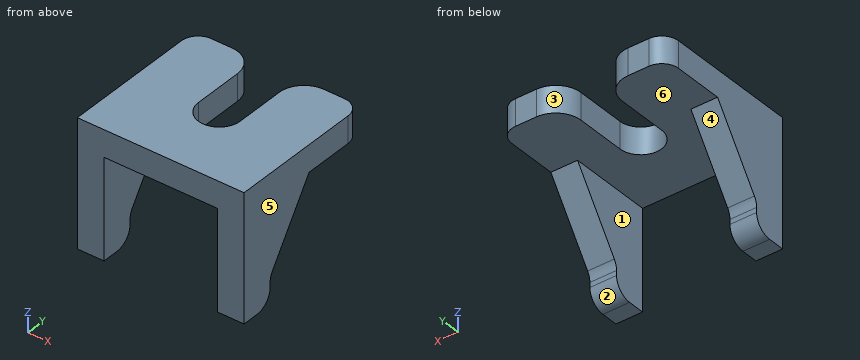
```python
from build123d import *

# Parameters (mm, degrees)
PAD006_DEPTH            = 1.6
PAD007_DEPTH            = 1.6
LINEARPATTERN009_COUNT  = 2
LINEARPATTERN009_PITCH  = 8.4
FILLET008_R             = 1
FILLET009_R             = 1
FILLET035_R             = 1
FILLET036_R             = 1.5
BODY003_PLACEMENT_ANGLE = 90


with BuildPart() as part:
    # Sketch110 → Pad006 (new body)
    with BuildSketch(Plane.XY):
        with BuildLine():
            Line((-4.5, 5), (4.5, 5))
            Line((4.5, 5), (4.5, 1.25))
            Line((0, 1.25), (4.5, 1.25))
            ThreePointArc((0, 1.25), (-1.25, 0), (0, -1.25))
            Line((4.5, -1.25), (0, -1.25))
            Line((4.5, -1.25), (4.5, -5))
            Line((4.5, -5), (-4.5, -5))
            Line((-4.5, -5), (-4.5, 5))
        make_face()
    extrude(amount=PAD006_DEPTH)

    # Sketch111 (on DatumPlane) → Pad007 (join)
    with BuildSketch(Plane.XZ.offset(5)):
        Polygon((-4.5, 0), (-4.5, -6), (-2.5, -6), (-2.5, -4.4), (0.5, 0), align=None)
    pad007 = extrude(amount=-PAD007_DEPTH)

    # LinearPattern009: Pad007 ×2
    with Locations(*[(0, i * LINEARPATTERN009_PITCH, 0) for i in range(1, LINEARPATTERN009_COUNT)]):
        add(pad007)

    # Fillet008
    fillet008_edges = [part.edges().sort_by_distance(p)[0] for p in [
        (-2.5, -4.2, -6),
        (-2.5, 4.2, -6),
    ]]
    fillet(fillet008_edges, radius=FILLET008_R)

    # Fillet009
    fillet009_edges = [part.edges().sort_by_distance(p)[0] for p in [
        (-2.5, -4.2, -4.4),
        (-2.5, 4.2, -4.4),
    ]]
    fillet(fillet009_edges, radius=FILLET009_R)

    # Fillet035
    fillet035_edges = [part.edges().sort_by_distance(p)[0] for p in [
        (4.5, -5, 0.8),
        (4.5, 5, 0.8),
    ]]
    fillet(fillet035_edges, radius=FILLET035_R)

    # Fillet036
    fillet036_edges = [part.edges().sort_by_distance(p)[0] for p in [
        (4.5, -1.25, 0.8),
        (4.5, 1.25, 0.8),
    ]]
    fillet(fillet036_edges, radius=FILLET036_R)


with BuildPart() as part_1:
    # Body003 placement: moved
    add(part.part.moved(Location((-22.4, 32.5, 16.4))).rotate(Axis((-22.4, 32.5, 16.4), (0, 0, 1)), BODY003_PLACEMENT_ANGLE))


solid = part_1.part
```
Input: part model. Units: mm. Frame: model coordinates. Face numbers are marked on the shaded views. A direction names the side the tool comes from. Give positions to 0.01 mm unless a question says otherwise; leave off trailing zeros. Order: outer loops, then holes, each group sorted by start corner. A loop starts at its lowest first (then second) coordinate and runs counter-clockwise, first axis right, second up. Notation, with made-up numbers: M 85,-8.5 L 115,-8.5 A31 cw 115,22.5 Z; hole C -25.5,22 d5. An arc over 180 degrees is marked long. One line per question, with ' | ' between items.
1) Access query for the marked faces 1, 2 and 3. Directions: +Z, -Z, +X, -X, +Y, -Y. A direction counts if a zero-diameter tool reaches every point of the face in a straight line with its end or side. Return the directions, or none.
Filled in:
face 1: -Z, +Y, -Y | face 2: -Z, +X, -X, +Y | face 3: +Z, -Z, +Y
2) Section A-A on y = 33.5. Output: boundary loops of the cut face in (x, z), and give its area (3 significant figures).
Filled in:
outline: M -27.4,16.4 L -23.65,16.4 L -23.65,18 L -27.4,18 Z; M -21.15,16.4 L -17.4,16.4 L -17.4,18 L -21.15,18 Z | area: 12.0 mm2
3) Section D-D on y = 29.25. Output: boundary loops of the cut face in (x, z), and give its area (3 significant figures).
Filled in:
outline: M -27.4,10.43 L -25.8,10.43 L -25.8,16.4 L -19,16.4 L -19,10.43 L -17.4,10.43 L -17.4,18 L -27.4,18 Z | area: 35.1 mm2
4) Contact query for flat-ended pins moving along their axis: P1, Ø4, axis at x = -19.5, y = 34, coming from the -Z side; P2, Ø4, axis at y = 31, z = 13, coming from the -X side; P3, Ø3, axis at x = -24, z = 13.5, coming from the -Y side. Output: stop coordinate, or through.
Filled in:
P1: stops at z = 15.03 | P2: stops at x = -27.4 | P3: passes through
5) Draft query along X for the marked faces 4, 5 and 6. Return one class per face: pulls with the +X half, pulls with the -X half, needs draft (parallel to the pull), parting line crosses it, or undercut.
Filled in:
face 4: needs draft | face 5: pulls with the +X half | face 6: undercut
6) Ray query, L1, parallel to X at y = 30, z = 15; L2, parallel to Z at x = -20.25, y = 33; L3, parallel to X at y = 32.25, z = 17.5. Return the intervals inside material, ascending.
Filled in:
L1: x = -27.4 to -25.8, -19 to -17.4 | L2: z = 16.4 to 18 | L3: x = -27.4 to -23.62, -21.18 to -17.4
7) Section C-C on z = 17.25. Output: boundary loops of the cut face in (x, y).
Filled in:
outline: M -27.4,28 L -17.4,28 L -17.4,36 A1 ccw -18.4,37 L -19.65,37 A1.5 ccw -21.15,35.5 L -21.15,32.5 A1.25 cw -23.65,32.5 L -23.65,35.5 A1.5 ccw -25.15,37 L -26.4,37 A1 ccw -27.4,36 Z
8) Section B-B on z = 14. Output: boundary loops of the cut face in (x, y), and give its area (3 significant figures).
Filled in:
outline: M -27.4,28 L -25.8,28 L -25.8,31.36 L -27.4,31.36 Z; M -19,28 L -17.4,28 L -17.4,31.36 L -19,31.36 Z | area: 10.8 mm2
